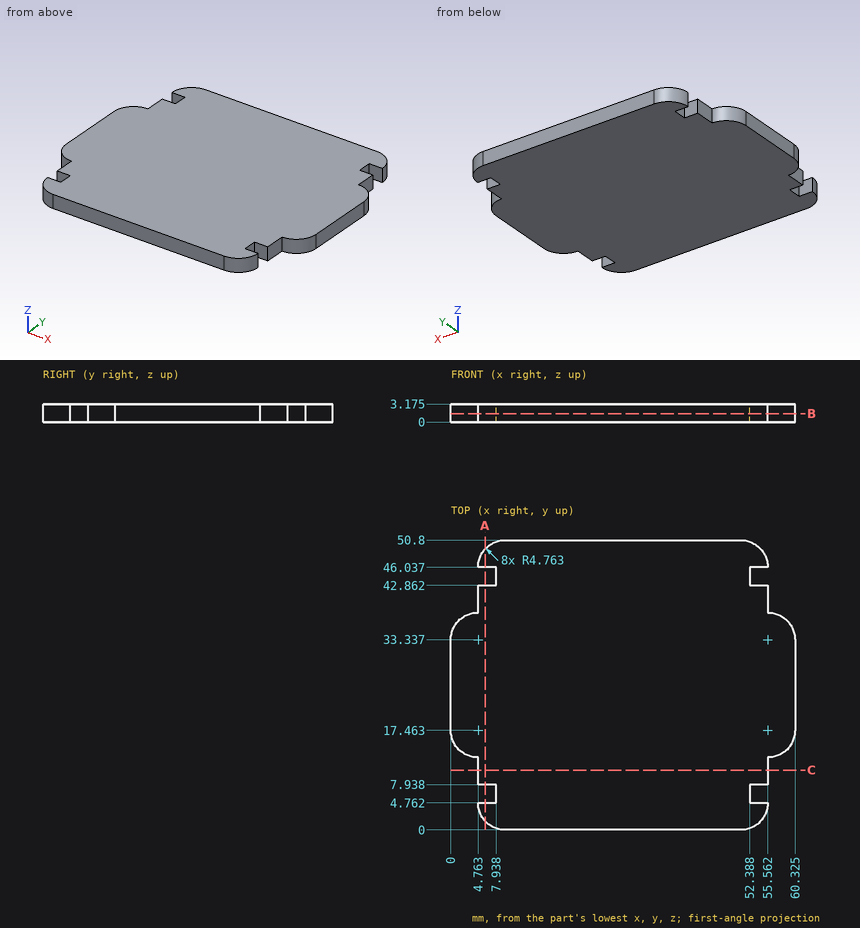
Here's the drawing with two shaded views (mm, measured from the low corner). I have some questions. Give positions to 0.01 mm unless a question says otherwise; leave off trailing zeros. Loops run counter-clockwise (first coordinate to the right, second up) from the corner with the lowest first, then second, coordinate; pieces in that order, holes last. Notation, with made-up numbers: M 35,35.5 L 73,35.5 A31 cw 73,60.5 Z; hole C 88,49.25 d11. An arc over 180 degrees is marked long. One line per item, written item: value. Start each with the question number.
1) If we section it at B-B, the plane z = 1.5: Write out the boundary of the cut face in (x, y) (1 decimal), and give its area (3 significant figures).
2) If we section it at C-C, the plane y = 10.5: Write out the boundary of the cut face in (x, z) (1 decimal), and give its area (3 significant figures).
3) If we section it at A-A, the plane x = 6: Write out the boundary of the cut face in (y, z) (1 decimal).
4) If I drill on line 1 (Y direction, x = 5.5, z = 1.95) (1 decimal); line 2 (X direction, y = 41.5, z = 1.35); line 3 (X direction, y = 44, z = 0.55), over which ranges is the centre line in solid material (lowest first)? Write a range as [from, to].
5) I'm going to push flat-ended pins straight in: pin 1 (1.6 mm diameter, centred on x = 6, z = 1, fed in from +Y); pin 2 (1.6 mm diameter, centred on x = 54, z = 2.5, fed in from +Y); pin 3 (1.6 mm diameter, centred on y = 6, z = 1.5, fed in from -X). Where does each tip first touch, or does it pass through?
Completed:
1. outline: M 0,17.5 A4.8 ccw 4.8,12.7 L 4.8,7.9 L 7.9,7.9 L 7.9,4.8 L 4.8,4.8 A4.8 ccw 9.5,0 L 50.8,0 A4.8 ccw 55.6,4.8 L 52.4,4.8 L 52.4,7.9 L 55.6,7.9 L 55.6,12.7 A4.8 ccw 60.3,17.5 L 60.3,33.3 A4.8 ccw 55.6,38.1 L 55.6,42.9 L 52.4,42.9 L 52.4,46 L 55.6,46 A4.8 ccw 50.8,50.8 L 9.5,50.8 A4.8 ccw 4.8,46 L 7.9,46 L 7.9,42.9 L 4.8,42.9 L 4.8,38.1 A4.8 ccw 0,33.3 Z
1. area: 2,740 mm^2
2. outline: M 4.8,0 L 55.6,0 L 55.6,3.2 L 4.8,3.2 Z
2. area: 161 mm^2
3. outline: M 1.6,0 L 4.8,0 L 4.8,3.2 L 1.6,3.2 Z; M 7.9,0 L 42.9,0 L 42.9,3.2 L 7.9,3.2 Z; M 46,0 L 49.2,0 L 49.2,3.2 L 46,3.2 Z
4. line 1: y = [2.2, 4.8], [7.9, 42.9], [46, 48.6]
4. line 2: x = [4.76, 55.56]
4. line 3: x = [7.94, 52.39]
5. pin 1: stops at y = 49.94
5. pin 2: stops at y = 50.15
5. pin 3: stops at x = 7.94
